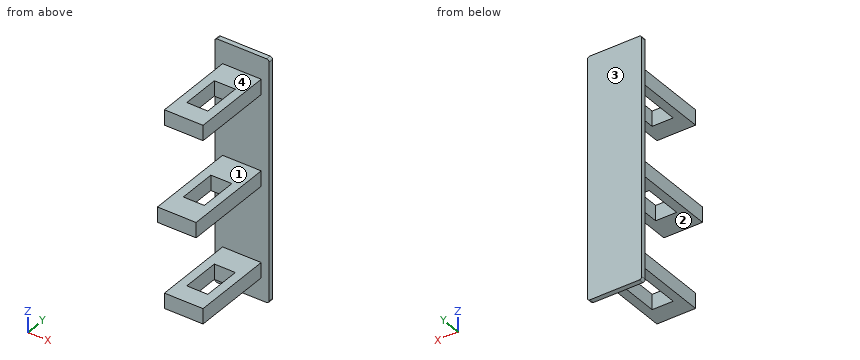
Autodesk Inventor part; units mm, degrees
ref_plane "to_body_XY" through (0, 0, 0) normal (0, 1, 0) x (1, 0, 0)
ref_plane "to_body_YZ" through (0, 0, 0) normal (1, 0, 0) x (0, 0, -1)
ref_plane "to_body_ZX" through (0, 0, 0) normal (0, 0, -1) x (0, 1, 0)
sketch "Sketch_1" plane through (0, 0, 0) normal (0, 1, 0) x (-1, 0, 0)
  line L0 (1.4097, -6.1214) -> (1.4097, 6.1214)
  arc A0 (1.4097, 6.1214) -> (1.2827, 6.2484) centre (1.2827, 6.1214) ccw
  line L1 (1.2827, 6.2484) -> (-1.2827, 6.2484)
  arc A1 (-1.2827, 6.2484) -> (-1.4097, 6.1214) centre (-1.2827, 6.1214) ccw
  line L2 (-1.4097, 6.1214) -> (-1.4097, -6.1214)
  arc A2 (-1.4097, -6.1214) -> (-1.2827, -6.2484) centre (-1.2827, -6.1214) ccw
  line L3 (-1.2827, -6.2484) -> (1.2827, -6.2484)
  arc A3 (1.2827, -6.2484) -> (1.4097, -6.1214) centre (1.2827, -6.1214) ccw
extrude "Extrusion1" add sketch "Sketch_1" along normal blind 0.254
sketch "Sketch_2" plane through (0, 0, -4.699) normal (0, 0, 1) x (1, 0, 0)
  line L0 (-1.0033, 0) -> (-1.0033, -4.2418)
  line L1 (-1.0033, -4.2418) -> (1.0033, -4.2418)
  line L2 (1.0033, -4.2418) -> (1.0033, 0)
  line L3 (1.0033, 0) -> (-1.0033, 0)
  line L4 (-0.5461, -1.2446) -> (-0.5461, -3.2512)
  line L5 (-0.5461, -3.2512) -> (0.5461, -3.2512)
  line L6 (0.5461, -3.2512) -> (0.5461, -1.2446)
  line L7 (0.5461, -1.2446) -> (-0.5461, -1.2446)
extrude "Extrusion2" add sketch "Sketch_2" along normal mid plane 0.7874
sketch "Sketch_3" plane through (0, 0, 4.699) normal (0, 0, 1) x (1, 0, 0)
  line L0 (-1.0033, 0) -> (-1.0033, -4.2418)
  line L1 (-1.0033, -4.2418) -> (1.0033, -4.2418)
  line L2 (1.0033, -4.2418) -> (1.0033, 0)
  line L3 (1.0033, 0) -> (-1.0033, 0)
  line L4 (-0.5461, -1.2446) -> (-0.5461, -3.2512)
  line L5 (-0.5461, -3.2512) -> (0.5461, -3.2512)
  line L6 (0.5461, -3.2512) -> (0.5461, -1.2446)
  line L7 (0.5461, -1.2446) -> (-0.5461, -1.2446)
extrude "Extrusion3" add sketch "Sketch_3" along normal mid plane 0.7874
sketch "Sketch_4" plane through (0, 0, 0) normal (0, 0, 1) x (1, 0, 0)
  line L0 (-1.0033, 0) -> (-1.0033, -4.7498)
  line L1 (-1.0033, -4.7498) -> (1.0033, -4.7498)
  line L2 (1.0033, -4.7498) -> (1.0033, 0)
  line L3 (1.0033, 0) -> (-1.0033, 0)
  line L4 (-0.5461, -1.4986) -> (-0.5461, -3.5052)
  line L5 (-0.5461, -3.5052) -> (0.5461, -3.5052)
  line L6 (0.5461, -3.5052) -> (0.5461, -1.4986)
  line L7 (0.5461, -1.4986) -> (-0.5461, -1.4986)
extrude "Extrusion4" add sketch "Sketch_4" along normal mid plane 0.7874
ref_plane "to_body_XY" through (0, 0, 0) normal (0, 1, 0) x (1, 0, 0)
ref_plane "to_body_YZ" through (0, 0, 0) normal (1, 0, 0) x (0, 0, -1)
ref_plane "to_body_ZX" through (0, 0, 0) normal (0, 0, -1) x (0, 1, 0)
properties part number "MB2011W01-terminals"
Can you work these out from the model? Positions are in its coordinate system, mm. Face numbers are marked on the shaded views. Round coordinates to 2 decimals unless told otherwise and drop trailing zeros. Loops run counter-clockwise (first coordinate to the right, second up) from the corner with the lowest first, then second, coordinate; pieces in that order, holes last. Notation, with made-up numbers: M -22,34.5 L 18,34.5 A33 ccw 18,67.5 Z; hole C 10,1 d5. An arc over 180 degrees is marked long. Write item = value, one per line. Start each with the question number.
(1) I need wall thicknesses on line 1 along Z through (x, y) = (-0.85, -3.25); line 2 along X through (y, z) = (-0.05, -4.5); line 3 along Y through (x, z) = (0.9, -0.5). Which ranges of each line are inside material? Lowest first, please.
(2) If we mould it in two halves opening along Z, with no side actions, what happens to the marked faces 1, 2, 3 and 4? For each: released by +Z, released by -Z, zero draft, split by the parting line, or undercut.
(3) Suppose I cut it at D-D on z = 0.25. Write out the boundary of the cut face in (x, y).
(4) I'm going to push flat-ended pins straight in: P1, Ø0.9, axis at y = -2.5, z = -5, coming from the -X side; P2, Ø0.6, axis at x = 0, y = -1, coming from the +Z side; P3, Ø0.6, axis at x = 0, z = 5, coming from the -Y side. Where does each tip first touch, or does it pass through?
(5) Suppose I cut it at B-B on y = -3.85. Write out the boundary of the cut face in (x, z).
(6) Suppose I cut it at C-C on y = -2.4. Write out the boundary of the cut face in (x, z).
(7) Suppose I cut it at A-A on x = 0.1. Write out the boundary of the cut face in (y, z), plus the area to 3 significant figures.
Answer block:
q1.line_1 = -5.09 to -4.31, -0.39 to 0.39, 4.31 to 5.09
q1.line_2 = -1 to 1
q1.line_3 = 0 to 0.25
q2.face_1 = undercut
q2.face_2 = undercut
q2.face_3 = zero draft
q2.face_4 = released by +Z
q3.outline = M -1.41,0 L -1,0 L -1,-4.75 L 1,-4.75 L 1,0 L 1.41,0 L 1.41,0.25 L -1.41,0.25 Z; hole M -0.55,-3.51 L 0.55,-3.51 L 0.55,-1.5 L -0.55,-1.5 Z
q4.P1 = -1
q4.P2 = 5.09
q4.P3 = -4.24
q5.outline = M -1,-5.09 L 1,-5.09 L 1,-4.31 L -1,-4.31 Z; M -1,-0.39 L 1,-0.39 L 1,0.39 L -1,0.39 Z; M -1,4.31 L 1,4.31 L 1,5.09 L -1,5.09 Z
q6.outline = M -1,-5.09 L -0.55,-5.09 L -0.55,-4.31 L -1,-4.31 Z; M -1,-0.39 L -0.55,-0.39 L -0.55,0.39 L -1,0.39 Z; M -1,4.31 L -0.55,4.31 L -0.55,5.09 L -1,5.09 Z; M 0.55,-5.09 L 1,-5.09 L 1,-4.31 L 0.55,-4.31 Z; M 0.55,-0.39 L 1,-0.39 L 1,0.39 L 0.55,0.39 Z; M 0.55,4.31 L 1,4.31 L 1,5.09 L 0.55,5.09 Z
q7.outline = M -4.75,-0.39 L -3.51,-0.39 L -3.51,0.39 L -4.75,0.39 Z; M -4.24,-5.09 L -3.25,-5.09 L -3.25,-4.31 L -4.24,-4.31 Z; M -4.24,4.31 L -3.25,4.31 L -3.25,5.09 L -4.24,5.09 Z; M -1.5,-0.39 L 0,-0.39 L 0,-4.31 L -1.24,-4.31 L -1.24,-5.09 L 0,-5.09 L 0,-6.25 L 0.25,-6.25 L 0.25,6.25 L 0,6.25 L 0,5.09 L -1.24,5.09 L -1.24,4.31 L 0,4.31 L 0,0.39 L -1.5,0.39 Z
q7.area = 8.85 mm²
